from build123d import *

# Parameters (mm, degrees)
F1_R     = 3.4925
F1_R_2   = 1.905
F2_DEPTH = 2.54
F1_R_3   = 1.651
F3_DEPTH = 7.62
F4_R     = 5.07999


# Not quite as in the source:
# - a fillet or chamfer is up to 0.001 mm smaller than in the source, because OpenCascade refuses the exact size


with BuildPart() as f2:
    # F1 (on Top) → F2 (new body)
    with BuildSketch(Plane.XY):
        with BuildLine():
            ThreePointArc((25.4, -22.5425), (21.9075, -19.05), (25.4, -15.5575))
            Line((25.4, -15.5575), (25.4, 5.3975))
            ThreePointArc((25.4, 5.3975), (21.9075, 8.89), (25.4, 12.3825))
            Line((25.4, 12.3825), (25.4, 14.9225))
            Line((25.4, 14.9225), (25.4, 28.575))
            Line((25.4, 28.575), (-32.7025, 28.575))
            Line((-32.7025, 28.575), (-32.7025, -30.1625))
            Line((-32.7025, -30.1625), (25.4, -30.1625))
            Line((25.4, -30.1625), (25.4, -25.0825))
            Line((25.4, -25.0825), (25.4, -22.5425))
        make_face()
        with Locations((-26.67, -24.13)):
            Circle(F1_R, mode=Mode.SUBTRACT)
        with Locations((-25.4, 24.13)):
            Circle(F1_R_2, mode=Mode.SUBTRACT)
        with BuildLine():
            ThreePointArc((25.4, -15.5575), (27.8695704333, -16.5804295667), (28.8925, -19.05))
            ThreePointArc((28.8925, -19.05), (27.8695704333, -21.5195704333), (25.4, -22.5425))
            Line((25.4, -22.5425), (25.4, -25.0825))
            Line((25.4, -25.0825), (31.4325, -25.0825))
            Line((31.4325, -25.0825), (31.4325, 14.9225))
            Line((31.4325, 14.9225), (25.4, 14.9225))
            Line((25.4, 14.9225), (25.4, 12.3825))
            ThreePointArc((25.4, 12.3825), (27.8695704333, 11.3595704333), (28.8925, 8.89))
            ThreePointArc((28.8925, 8.89), (27.8695704333, 6.4204295667), (25.4, 5.3975))
            Line((25.4, 5.3975), (25.4, -15.5575))
        make_face()
    extrude(amount=F2_DEPTH)

    # F1 (on Top) → F3 (join)
    with BuildSketch(Plane.XY):
        with Locations((-26.67, -24.13)):
            Circle(F1_R)
        with Locations((-26.67, -24.13)):
            Circle(F1_R_3, mode=Mode.SUBTRACT)
        with Locations((-25.4, 24.13)):
            Circle(F1_R_2)
        with BuildLine():
            ThreePointArc((25.4, 12.3825), (21.9075, 8.89), (25.4, 5.3975))
            Line((25.4, 5.3975), (25.4, 7.239))
            ThreePointArc((25.4, 7.239), (23.749, 8.89), (25.4, 10.541))
            Line((25.4, 10.541), (25.4, 12.3825))
        make_face()
        with BuildLine():
            Line((25.4, 7.239), (25.4, 5.3975))
            ThreePointArc((25.4, 5.3975), (27.8695704333, 6.4204295667), (28.8925, 8.89))
            ThreePointArc((28.8925, 8.89), (27.8695704333, 11.3595704333), (25.4, 12.3825))
            Line((25.4, 12.3825), (25.4, 10.541))
            ThreePointArc((25.4, 10.541), (26.5674332957, 10.0574332957), (27.051, 8.89))
            ThreePointArc((27.051, 8.89), (26.5674332957, 7.7225667043), (25.4, 7.239))
        make_face()
        with BuildLine():
            Line((25.4, -17.399), (25.4, -15.5575))
            ThreePointArc((25.4, -15.5575), (21.9075, -19.05), (25.4, -22.5425))
            Line((25.4, -22.5425), (25.4, -20.701))
            ThreePointArc((25.4, -20.701), (23.749, -19.05), (25.4, -17.399))
        make_face()
        with BuildLine():
            ThreePointArc((25.4, -22.5425), (27.8695704333, -21.5195704333), (28.8925, -19.05))
            ThreePointArc((28.8925, -19.05), (27.8695704333, -16.5804295667), (25.4, -15.5575))
            Line((25.4, -15.5575), (25.4, -17.399))
            ThreePointArc((25.4, -17.399), (26.5674332957, -17.8825667043), (27.051, -19.05))
            ThreePointArc((27.051, -19.05), (26.5674332957, -20.2174332957), (25.4, -20.701))
            Line((25.4, -20.701), (25.4, -22.5425))
        make_face()
    extrude(amount=F3_DEPTH)

    # F4 (radius 5.08 in the source; OpenCascade refuses exactly that, so slightly less here)
    f4_edges = [f2.edges().sort_by_distance(p)[0] for p in [
        (-32.7025, -30.1625, 1.27),
        (25.4, -30.1625, 1.27),
        (31.4325, -25.0825, 1.27),
        (31.4325, 14.9225, 1.27),
        (25.4, 28.575, 1.27),
        (-32.7025, 28.575, 1.27),
    ]]
    fillet(f4_edges, radius=F4_R)


solid = f2.part
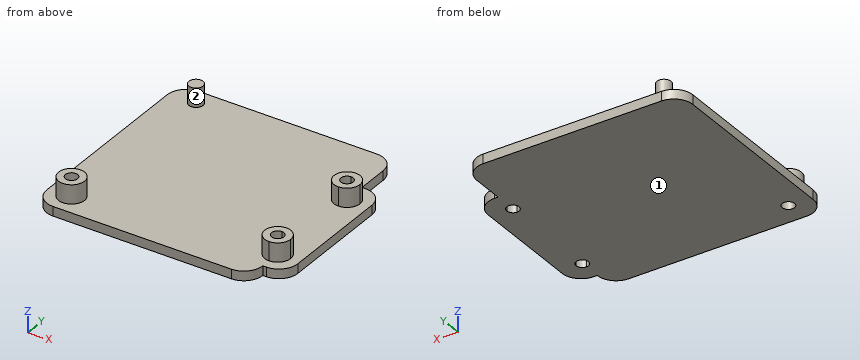
Input: part model. Units: mm. Frame: model coordinates. Face numbers are marked on the shaded views. Coordinates: 2 decimals unless noted, no trailing zeros. Order: outer loops, then holes, each group sorted by start corner. A loop starts at its lowest first (then second) coordinate and runs counter-clockwise, first axis right, second up. Notation, with made-up numbers: M 24.5,-17 L 31.5,-17 A8 ccw 31.5,-6 Z; hole C 27.25,89 d8. An arc over 180 degrees is marked long. Answer in a Markdown table with one row per item.
(1) Section query A-A, the plane z = 6.25. Give the number of separate pieces and of enclosed holes in the cut face, plus the area to 3 significant figures.
Numbers:
| item | result |
|---|---|
| separate pieces | 4 |
| enclosed holes | 3 |
| area | 101 mm^2 |
(2) Material intervals for line 1 (Y direction, x = -26.67, z = 3.75); line 2 (Z direction, x = -11.5, y = -24); line 3 (Y direction, x = -26.67, z = 2) (1 decimal), sorted ascending. Write a range as [from, to].
Numbers:
| item | result |
|---|---|
| line 1 | y = [-27.62, -25.78], [-22.48, -20.64], [22.71, 25.55] |
| line 2 | z = [0, 2.54] |
| line 3 | y = [-30.2, -25.8], [-22.5, 28.6] |
(3) Section query D-D, the plane y = -11. Output: boundary loops of the cut face in (x, z).
Numbers:
| item | result |
|---|---|
| outline | M -32.7,0 L 31.43,0 L 31.43,2.54 L -32.7,2.54 Z |
(4) Section query C-C, the plane x = 5. Output: boundary loops of the cut face in (y, z) (1 decimal), plus the area to 3 significant figures.
Numbers:
| item | result |
|---|---|
| outline | M -30.2,0 L 28.6,0 L 28.6,2.5 L -30.2,2.5 Z |
| area | 149 mm^2 |
(5) Section query B-B, the plane y = -24.13. Output: boundary loops of the cut face in (x, z), plus the area to 3 significant figures.
Numbers:
| item | result |
|---|---|
| outline | M -32.7,0 L -28.32,0 L -28.32,7.62 L -30.16,7.62 L -30.16,2.54 L -32.7,2.54 Z; M -25.02,0 L 29.31,0 L 29.31,2.54 L -23.18,2.54 L -23.18,7.62 L -25.02,7.62 Z |
| area | 168 mm^2 |
(6) Contact query for flat-ended pins moving along their axis: pin 1 Ø0.8 at (x, z) = (26, 1) entering from +Y; pin 2 Ø1.5 at (x, y) = (20, -15.5) entering from +Z; pin 3 Ø2 at (y, z) = (17, 1.5) entering from +X. Output: stop coordinate, or through.
Numbers:
| item | result |
|---|---|
| pin 1 | stops at y = 14.92 |
| pin 2 | stops at z = 2.54 |
| pin 3 | stops at x = 25.4 |
(7) Draft query along Y for the marked faces 1 and 2. Return one class per face: pulls with the +Y half, pulls with the -Y half, needs draft (parallel to the pull), parting line crosses it, or undercut.
Numbers:
| item | result |
|---|---|
| face 1 | needs draft |
| face 2 | undercut |
